from build123d import *

# Parameters (mm, degrees)
EXTRUDE_1_DEPTH     = 3
SKETCH_2_R          = 1.5
CUT_EXTRUDE_1_DEPTH = 3
FILLET_1_R          = 3
SKETCH_3_R          = 1.5
CUT_EXTRUDE_2_DEPTH = 10
SKETCH_4_W          = 80
SKETCH_4_H          = 5
EXTRUDE_2_DEPTH     = 3
FILLET_2_R          = 5


with BuildPart() as part:
    # 草图1 → 凸台-拉伸1 (new body)
    with BuildSketch(Plane(origin=(0, 0, 0), x_dir=(1, 0, 0), z_dir=(0, 1, 0))):
        Polygon((-40, 1), (-40, -25), (40, -25), (40, 1), (32, 1), (32, 25), (-32, 25), (-32, 1), align=None)
    extrude(amount=EXTRUDE_1_DEPTH)

    # 草图2 → 切除-拉伸1 (cut)
    with BuildSketch(Plane(origin=(0, 3, 0), x_dir=(1, 0, 0), z_dir=(0, 1, 0))):
        with Locations(Location((-32, -19, 0), (0, 0, 270))):
            Circle(SKETCH_2_R)
        with Locations(Location((32, -19, 0), (0, 0, 90))):
            Circle(SKETCH_2_R)
        with Locations(Location((-27, 19, 0), (0, 0, 270))):
            Circle(SKETCH_2_R)
        with Locations(Location((27, 19, 0), (0, 0, 90))):
            Circle(SKETCH_2_R)
    extrude(amount=-CUT_EXTRUDE_1_DEPTH, mode=Mode.SUBTRACT)

    # 圆角1
    fillet_1_edges = [part.edges().sort_by_distance(p)[0] for p in [
        (32, 1.5, -1),
        (40, 1.5, -1),
        (-40, 1.5, -1),
        (-32, 1.5, -1),
    ]]
    fillet(fillet_1_edges, radius=FILLET_1_R)

    # 草图3 → 切除-拉伸2 (cut)
    with BuildSketch(Plane(origin=(0, 3, 0), x_dir=(1, 0, 0), z_dir=(0, 1, 0))):
        with Locations(Location((-15, 1, 0), (0, 0, 270))):
            Circle(SKETCH_3_R)
        with Locations(Location((-15, -23, 0), (0, 0, 270))):
            Circle(SKETCH_3_R)
        with Locations(Location((15, -23, 0), (0, 0, 270))):
            Circle(SKETCH_3_R)
        with Locations(Location((15, 1, 0), (0, 0, 270))):
            Circle(SKETCH_3_R)
    extrude(amount=-CUT_EXTRUDE_2_DEPTH, mode=Mode.SUBTRACT)

    # 草图4 → 凸台-拉伸2 (add)
    with BuildSketch(Plane(origin=(0, 3, 0), x_dir=(1, 0, 0), z_dir=(0, 1, 0))):
        with Locations((0, -27.5)):
            Rectangle(SKETCH_4_W, SKETCH_4_H)
    extrude(amount=-EXTRUDE_2_DEPTH)

    # 圆角2
    fillet_2_edges = [part.edges().sort_by_distance(p)[0] for p in [
        (-32, 1.5, -25),
        (32, 1.5, -25),
        (40, 1.5, 30),
        (-40, 1.5, 30),
    ]]
    fillet(fillet_2_edges, radius=FILLET_2_R)


solid = part.part
CAD build for the part. Positions are in the model's coordinates, mm. A direction names the side the tool comes from. Give positions to 0.01 mm unless a question says otherwise; leave off trailing zeros. Loops run counter-clockwise (first coordinate to the right, second up) from the corner with the lowest first, then second, coordinate; pieces in that order, holes last. Notation, with made-up numbers: M 52,7 L 96,7 A22 ccw 96,27 Z; hole C 52,-18 d2. An arc over 180 degrees is marked long. One line per question, with ' | ' between items. Start each with the question number.
1. Flat gauge pins, fed straight in: pin 1 (0.9 mm diameter, centred on y = 1, z = -14, fed in from -X); pin 2 (0.6 mm diameter, centred on x = -36, y = 1.5, fed in from -Z). Where does each tip first touch, or does it go through?
2. Saw through at C-C on y = 1.5. State how many separate pieces and enclosed holes the cut face has, plus the area to 3 significant figures.
3. Saw through at B-B on x = -15. Give the cut face in (y, z).
4. Two-plate mould, pull along X, no slides. Class faces 1 (the face through (0, 1, -25)), 2 (the face through (31.93, 1.52, 20.5)), 3 (the face through (-40, 2, 14)): pulls with the +X half, pulls with the -X half, needs draft (parallel to the pull), parting line crosses it, or undercut.
5. Saw through at D-D on z = -12.5. Give the cut face in (x, y).
6. Probe L1, parallel to X at y = 0.7, z = -19; L2, parallel to X at y = 1.65, z = -14; L3, parallel to X at y = 0.9, z = 1.5. List the from-to ranges inside material, lowest first. Write a range as from..to.
7. 3-axis set-ups, long thin cutter, end or side, ignore diameter. For faces 4 (the face through (32, 1, -12)), 5 (the face through (15.07, 1.52, 21.5)), 6 (the face through (-36, 1, -1)): which of +Z, -Z, +X, -X, +Y, -Y reach the whole face in a straight line?
8. Saw through at A-A on z = -19. Give the cut face in (x, y).
Result sheet:
1) pin 1: stops at x = -32 | pin 2: stops at z = -1
2) separate pieces: 1 | enclosed holes: 8 | area: 3,940 mm^2
3) outline: M 0,-25 L 3,-25 L 3,-2.5 L 0,-2.5 Z; M 0,0.5 L 3,0.5 L 3,21.5 L 0,21.5 Z; M 0,24.5 L 3,24.5 L 3,30 L 0,30 Z
4) face 1: needs draft | face 2: undercut | face 3: pulls with the -X half
5) outline: M -32,0 L 32,0 L 32,3 L -32,3 Z
6) L1: x = -32..-28.5, -25.5..25.5, 28.5..32 | L2: x = -32..32 | L3: x = -39.96..39.96
7) face 4: -Z, +X, +Y, -Y | face 5: +Y, -Y | face 6: -Z, -X, +Y, -Y
8) outline: M -32,0 L -28.5,0 L -28.5,3 L -32,3 Z; M -25.5,0 L 25.5,0 L 25.5,3 L -25.5,3 Z; M 28.5,0 L 32,0 L 32,3 L 28.5,3 Z
